Work out the finished part from the listing and answer in its coordinate system (mm). A direction names the side the tool comes from. Round coordinates to 2 decimals unless told otherwise and drop trailing zeros. Write each loop counter-clockwise with the first axis right and the second up, starting at its lowest first coordinate (ties: lowest second). Pieces come first, ordered by that corner, then holes. Notation, with made-up numbers: M 68,23 L 72,23 A29 cw 72,60 Z; hole C 89.5,-10.5 d7. An arc over 180 degrees is marked long. One line per item, written item: value. Start each with the question number.
Q1. Consider probe 1 along X at (y, z) = (4.75, -71.5); probe 2 along X at (y, z) = (9.25, -69); probe 3 along Z at (x, y) = (-54.5, 1.75). Determine where each line is inside the solid, lowest interval first.
Q2. Find section D-D (x = -10). Write down the section's boundary in (y, z) (3 decimals).
Q3. A tool of negligible diameter and unlimited length cuts with its end or side. For faces 4 (the flat face through (-17.78, 9, -86)), 5 (the flat face through (-30, 3, 0)), 6 (the flat face through (-30, 3, -6.35)), 7 (the flat face through (-52, 3, -111.76)), 8 (the flat face through (-6, 0, -47)), from which of +Z, -Z, +X, -X, +Y, -Y can it reach the whole face along a straight path? Write none if from no direction.
Q4. Find section C-C (z = -3). Write down the section's boundary in (x, y) (3 decimals).
Q5. Given pin 1 Ø1.5 at (x, z) = (-53.5, -78.5) entering from -Y; pin 2 Ø3 at (y, z) = (2, -61.5) entering from +X; pin 3 Ø5 at (x, y) = (-47.5, 2.5) entering from +Z; pin 4 Ø4 at (y, z) = (4.5, -79.5) entering from -X, each flat-ended and moving along its own axis, determine where each tip first touches the part or whether it passes through.
Q6. Find section B-B (y = 4.5). Write down the section's boundary in (x, z), and give its area (3 significant figures).
Q7. Find section A-A (z = -88). Write down the section's boundary in (x, y) (3 decimals), and give its area (3 significant figures).
Q8. The mould has two halves that part along X. Classify faces 1 (the flat face through (-31, 12.7, -44)), 2 (the flat face through (-49, 3, -105.41)), 3 (the flat face through (-68.58, 8, -56)): released by +X, released by -X, zero draft, split by the parting line, or undercut.
Autodesk Inventor part; units mm, degrees
ref_plane "YZ Plane" through (0, 0, 0) normal (1, 0, 0) x (0, 1, 0)
ref_plane "XZ Plane" through (0, 0, 0) normal (0, 1, 0) x (-1, 0, 0)
ref_plane "XY Plane" through (0, 0, 0) normal (0, 0, 1) x (1, 0, 0)
sketch "Sketch1" plane through (0, 0, 0) normal (0, 1, 0) x (-1, 0, 0)
  line L0 (0, 0) -> (60.96, 0)
  line L1 (60.96, 0) -> (60.96, -111.76)
  line L2 (60.96, -111.76) -> (0, -111.76)
  line L3 (0, -111.76) -> (0, 0)
  dimension "d0" = 60.96
  dimension "d1" = 111.76
extrude "Extrusion1" add sketch "Sketch1" along normal blind 6.35
sketch "Sketch2" plane through (0, 6.35, 0) normal (0, 1, 0) x (1, 0, 0)
  line L0 (-60.96, 0) -> (0, 0)
  line L1 (0, 0) -> (0, 111.76)
  line L2 (0, 111.76) -> (-60.96, 111.76)
  line L3 (-60.96, 111.76) -> (-60.96, 0)
  line L4 (7.62, -7.62) -> (-68.58, -7.62)
  line L5 (-68.58, -7.62) -> (-68.58, 119.38)
  line L6 (-68.58, 119.38) -> (7.62, 119.38)
  line L7 (7.62, 119.38) -> (7.62, -7.62)
  dimension "d4" = 7.62
extrude "Extrusion2" add sketch "Sketch2" along normal blind 6.35 contours L3 L2 L1 L0 | L4 L5 L6 L7
sketch "Sketch3" plane through (7.62, 6.35, 7.62) normal (1, 0, 0) x (0, 0, -1)
  line L0 (127, 0) -> (127, 6.35)
  line L1 (127, 0) -> (129.0632, 6.35)
  line L2 (127, 0) -> (136.5189, 0) construction
  line L3 (127, 6.35) -> (129.0632, 6.35)
  line L4 (0, 0) -> (0, 6.35)
  line L5 (0, 0) -> (2.0632, 6.35)
  line L6 (127, 6.35) -> (0, 6.35)
  line L7 (127, 0) -> (0, 0)
  line L8 (127, 0) -> (127, 6.35)
  line L9 (0, 6.35) -> (127, 6.35)
  line L10 (0, 0) -> (0, 6.35)
  point P0 (7.62, -6.35)
  dimension "d7" = 72
extrude "Extrusion3" add sketch "Sketch3" against normal blind 76.2 contours L0 L3 L1 | L4 L6 L5
sketch "Sketch4" plane through (7.62, 6.35, 7.62) normal (1, 0, 0) x (0, 0, -1)
  line L0 (0, 0) -> (2.0632, 6.35)
  line L1 (0, 0) -> (11.0448, 0) construction
  line L2 (0, 0) -> (0, 6.35)
  line L3 (0, 6.35) -> (129.0632, 6.35)
  point P0 (7.62, -6.35)
  dimension "d10" = 72
extrude "Extrusion4" cut sketch "Sketch4" against normal through all
fillet "Fillet2" radius 3.175 8 edges at (-68.58, 12.7, -57.9432) (-30.48, 12.7, -121.4432) (7.62, 12.7, -57.9432) (-68.58, 9.525, -120.4116) (7.62, 9.525, -120.4116) (7.62, 9.525, 6.5884) (-68.58, 9.525, 6.5884) (-30.48, 12.7, 5.5568)
sketch "Sketch5" plane through (0, 0, 0) normal (0, -1, 0) x (1, 0, 0)
  line L0 (0, 0) -> (-60.96, 0)
  line L1 (-60.96, 0) -> (-60.96, -111.76)
  line L2 (-60.96, -111.76) -> (0, -111.76)
  line L3 (0, -111.76) -> (0, 0)
  line L4 (-6.35, -6.35) -> (-54.61, -6.35)
  line L5 (-54.61, -6.35) -> (-54.61, -105.41)
  line L6 (-54.61, -105.41) -> (-6.35, -105.41)
  line L7 (-6.35, -105.41) -> (-6.35, -6.35)
  dimension "d16" = 6.35
extrude "Extrusion5" cut sketch "Sketch5" against normal blind 6.35 contours L7 L6 L5 L4
sketch "Sketch6" plane through (0, 0, 0) normal (0, -1, 0) x (1, 0, 0)
  line L0 (-60.96, -111.76) -> (0, -111.76)
  line L1 (-30.48, -111.76) -> (-17.78, -111.76)
  line L2 (-6.35, -105.41) -> (-54.61, -105.41)
  line L3 (-17.78, -111.76) -> (-43.18, -111.76)
  line L4 (-43.18, -111.76) -> (-43.18, -105.41)
  line L5 (-43.18, -105.41) -> (-17.78, -105.41)
  line L6 (-17.78, -105.41) -> (-17.78, -111.76)
  point P0 (0, 0)
  dimension "d19" = 12.7
  dimension "d20" = 25.4
extrude "Extrusion6" cut sketch "Sketch6" against normal blind 6.35
sketch "Sketch7" plane through (0, 6.35, 0) normal (0, -1, 0) x (1, 0, 0)
  line L0 (-17.78, -105.41) -> (-17.78, -111.76)
  line L1 (-17.78, -111.76) -> (-43.18, -111.76)
  line L2 (-43.18, -111.76) -> (-43.18, -142.1145)
  line L3 (-43.18, -142.1145) -> (-17.78, -142.1145)
  line L4 (-17.78, -142.1145) -> (-17.78, -111.76)
  line L5 (-43.18, -142.1145) -> (-17.78, -142.1145)
  line L6 (-17.78, -142.1145) -> (-17.78, -89.8971)
  line L7 (-17.78, -89.8971) -> (-43.18, -89.8971)
  line L8 (-43.18, -89.8971) -> (-43.18, -142.1145)
  point P0 (0, 0)
extrude "Extrusion7" cut sketch "Sketch7" against normal blind 25.4
sketch "Sketch8" plane through (0, 6.35, 0) normal (0, -1, 0) x (1, 0, 0)
  line L0 (-43.18, -89.8971) -> (-17.78, -89.8971)
  line L1 (-17.78, -89.8971) -> (-43.18, -89.8971)
  line L2 (-43.18, -89.8971) -> (-43.18, -52.3331)
  line L3 (-43.18, -52.3331) -> (-17.78, -52.3331)
  line L4 (-17.78, -52.3331) -> (-17.78, -89.8971)
  point P0 (0, 0)
extrude "Extrusion8" cut sketch "Sketch8" against normal blind 25.4
properties part number "Lid"
The answers:
1. probe 1: -60.96 to -54.61, -6.35 to 0
1. probe 2: -68.58 to -43.18, -17.78 to 7.62
1. probe 3: -111.76 to -105.41, -6.35 to 0
2. outline: M 0,-111.76 L 6.35,-111.76 L 6.35,-119.38 L 8.544,-120.093 A3.175 ccw 12.7,-117.073 L 12.7,3.25 A3.175 ccw 10.506,6.27 L 6.35,7.62 L 6.35,0 L 0,0 L 0,-6.35 L 6.35,-6.35 L 6.35,-105.41 L 0,-105.41 Z
3. face 4: -Z, +Y, -Y
3. face 5: +Z, +X, -X, -Y
3. face 6: -Y
3. face 7: -Z, +X, -X, -Y
3. face 8: +Z, -Z, +X, -X, -Y
4. outline: M -68.58,6.35 L -60.96,6.35 L -60.96,0 L 0,0 L 0,6.35 L 7.62,6.35 L 7.62,9.525 A3.175 ccw 4.445,12.7 L -65.405,12.7 A3.175 ccw -68.58,9.525 Z
5. pin 1: y = 6.35
5. pin 2: x = 0
5. pin 3: z = 0
5. pin 4: x = -68.58
6. outline: M -60.96,-111.76 L -43.18,-111.76 L -43.18,-105.41 L -54.61,-105.41 L -54.61,-6.35 L -6.35,-6.35 L -6.35,-105.41 L -17.78,-105.41 L -17.78,-111.76 L 0,-111.76 L 0,0 L -60.96,0 Z
6. area: 1,870 mm2
7. outline: M -68.58,6.35 L -60.96,6.35 L -60.96,0 L -54.61,0 L -54.61,6.35 L -43.18,6.35 L -43.18,12.7 L -65.405,12.7 A3.175 ccw -68.58,9.525 Z; M -17.78,6.35 L -6.35,6.35 L -6.35,0 L 0,0 L 0,6.35 L 7.62,6.35 L 7.62,9.525 A3.175 ccw 4.445,12.7 L -17.78,12.7 Z
7. area: 399 mm2
8. face 1: zero draft
8. face 2: undercut
8. face 3: released by -X
